Build history of the part. All positions in model axes, mm. A direction names the side the tool comes from. Round coordinates to 2 decimals unless told otherwise and drop trailing zeros. Write each loop counter-clockwise with the first axis right and the second up, starting at its lowest first coordinate (ties: lowest second). Pieces come first, ordered by that corner, then holes. Notation, with made-up numbers: (4, -17) -> (21, -17) arc R32 ccw to (21, 21) -> close; hole circle Ø10 at (-10, 78.5). An arc over 180 degrees is marked (long way). Answer as CSV lines item,"result".
from build123d import *

# Parameters (mm, degrees)
F1_DEPTH = 170
F2_W     = 1060
F2_H     = 200
F3_DEPTH = 20
F4_R     = 5
F5_R     = 5
F6_R     = 5
F7_R     = 5


with BuildPart() as f1:
    # F0 (on Front) → F1 (new body)
    with BuildSketch(Plane.XZ):
        Polygon((500, 1010), (0, 1010), (-500, 1010), (-500, 0), (-300, 0), (-300, 700), (0, 700), (300, 700), (300, 0), (500, 0), align=None)
    extrude(amount=F1_DEPTH)

    # F2 (on face) → F3 (join)
    with BuildSketch(Plane.XY.offset(1010)):
        with Locations((0, -100)):
            Rectangle(F2_W, F2_H)
    extrude(amount=F3_DEPTH)

    # F4
    f4_edges = [f1.edges().sort_by_distance(p)[0] for p in [
        (0, -200, 1010),
    ]]
    fillet(f4_edges, radius=F4_R)

    # F5
    f5_edges = [f1.edges().sort_by_distance(p)[0] for p in [
        (0, -200, 1030),
    ]]
    fillet(f5_edges, radius=F5_R)

    # F6
    f6_edges = [f1.edges().sort_by_distance(p)[0] for p in [
        (530, -97.5, 1030),
    ]]
    fillet(f6_edges, radius=F6_R)

    # F7
    f7_edges = [f1.edges().sort_by_distance(p)[0] for p in [
        (-530, -97.5, 1030),
    ]]
    fillet(f7_edges, radius=F7_R)


solid = f1.part
1. Drop flat-ended pins along their axis: pin 1 Ø5 at (y, z) = (-55, 834) entering from +X; pin 2 Ø10 at (y, z) = (-116, 590) entering from -X; pin 3 Ø2 at (x, z) = (375.5, 564.5) entering from -Y. Give the stop position or say it passes through.
Results found:
pin 1,"stops at x = 500"
pin 2,"stops at x = -500"
pin 3,"stops at y = -170"
2. Mould opens along X. For faces 1 (the flat face through (500, -84, 498)), 2 (the flat face through (-2, -184, 1010)), 3 (the flat face through (-300, -84, 345)) say: +X half, -X half, draft (parallel to the pull), parting line (faces both ways), or undercut.
Results found:
face 1,"+X half"
face 2,"draft"
face 3,"undercut"
3. Cut at B-B, the plane x = 424. Write the cut outline in (y, z), then the cut area to 3 significant figures.
Results found:
outline,"(-200, 1015) arc R5 ccw to (-195, 1010) -> (-170, 1010) -> (-170, 0) -> (0, 0) -> (0, 1030) -> (-195, 1030) arc R5 ccw to (-200, 1025) -> close"
area,"176,000 mm2"
4. Which spindle directions (+Z, -Z, +X, -X, +Y, -Y) get a long thin tool onto all of the face, cutting with end or side? Do faces 4 (the flat face through (300, -84, 355)), 5 (the flat face through (-500, -84, 512)), 6 (the flat face through (-7, -170, 737)). Say none if no direction does.
Results found:
face 4,"-Z, +Y, -Y"
face 5,"-Z, -X, +Y, -Y"
face 6,"-Z, +X, -X, -Y"
5. Cut at D-D, the plane x = -46. Write the cut outline in (y, z).
Results found:
outline,"(-200, 1015) arc R5 ccw to (-195, 1010) -> (-170, 1010) -> (-170, 700) -> (0, 700) -> (0, 1030) -> (-195, 1030) arc R5 ccw to (-200, 1025) -> close"
6. Cut at A-A, the plane z = 415. Write the cut outline in (x, y), then the cut area to 3 significant figures.
Results found:
outline,"(-500, -170) -> (-300, -170) -> (-300, 0) -> (-500, 0) -> close; (300, -170) -> (500, -170) -> (500, 0) -> (300, 0) -> close"
area,"68,000 mm2"
7. Cut at C-C, the plane y = -26. Write the cut outline in (x, z), then the cut area to 3 significant figures.
Results found:
outline,"(-530, 1015) arc R5 ccw to (-525, 1010) -> (-500, 1010) -> (-500, 0) -> (-300, 0) -> (-300, 700) -> (300, 700) -> (300, 0) -> (500, 0) -> (500, 1010) -> (525, 1010) arc R5 ccw to (530, 1015) -> (530, 1025) arc R5 ccw to (525, 1030) -> (-525, 1030) arc R5 ccw to (-530, 1025) -> close"
area,"611,000 mm2"
8. Probe line 1 along X through (y, z) = (-105, 301); line 2 along Y through (x, z) = (-479, 741); line 3 along Z through (x, y) = (48, -190). List the from-to ranges inside material, lowest first.
Results found:
line 1,"x = -500 to -300, 300 to 500"
line 2,"y = -170 to 0"
line 3,"z = 1010 to 1030"
